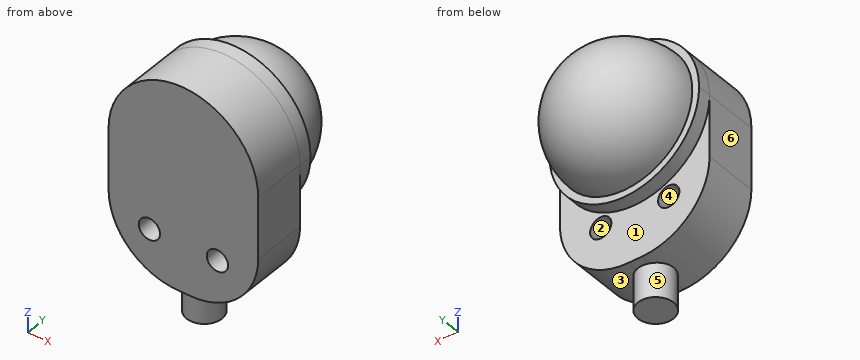
Autodesk Inventor part; units mm, degrees
ref_plane "Work Plane1" through (0, 0, 0) normal (1, 0, 0) x (0, 0, -1)
ref_plane "Work Plane2" through (0.5, 0, -9) normal (0, 0, -1) x (-1, 0, 0)
ref_plane "YZ Plane" through (0, 0, 0) normal (1, 0, 0) x (0, 1, 0)
sketch "Sketch1" plane through (0, 0, 0) normal (0, 1, 0) x (-1, 0, 0)
  arc A0 (5.5, 0) -> (-5.5, 0) centre (0, 0) ccw
  line L0 (5.5, 0) -> (5.5, -4.5)
  line L1 (-5.5, 0) -> (-5.5, -4.5)
  line L2 (-0.5, -9.5) -> (0.5, -9.5)
  arc A1 (-5.5, -4.5) -> (-0.5, -9.5) centre (-0.5, -4.5) ccw
  arc A2 (0.5, -9.5) -> (5.5, -4.5) centre (0.5, -4.5) ccw
  line L3 (0, 0) -> (0, -9.5) construction
  dimension "d0" = 11
  dimension "d1" = 15
  dimension "d2" = 5
extrude "Extrusion1" add sketch "Sketch1" along normal blind 4
sketch "Sketch2" plane through (0, 4, 0) normal (0, 1, 0) x (1, 0, 0)
  circle A0 centre (0, 0) radius 5.5
  arc A1 (-5.5, 0) -> (5.5, 0) centre (0, 0) ccw
extrude "Extrusion2" add sketch "Sketch2" along normal blind 1
ref_plane "Work Plane1" through (0, 0, 0) normal (1, 0, 0) x (0, 0, -1)
sketch "Sketch4" plane through (0, 0, 0) normal (1, 0, 0) x (0, 0, -1)
  line L0 (5.5, 5) -> (-5.5, 5)
  line L1 (0, 5) -> (0, 11.0328) construction
  arc A0 (5, 5) -> (0, 10) centre (0, 5) ccw
  line L2 (0, 10) -> (0, 5)
  line L3 (0, 5) -> (5, 5)
  point P0 (0, 0)
  dimension "d8" = 5
revolve "Revolution1" add sketch "Sketch4" angle 360 about axis through (0, 5, 0) along (0, 1, 0)
sketch "Sketch5" plane through (0, 0, 0) normal (0, -1, 0) x (1, 0, 0)
  line L0 (0, 0) -> (0, -9.4931) construction
  point P0 (2.5, -6)
  point P1 (-2.5, -6)
  dimension "d10" = 6
  dimension "d11" = 5
hole "Hole1" at (2.5, 0, -6) at (-2.5, 0, -6) direction (0, 1, 0) diameter 1.567 end through all
ref_plane "Work Plane2" through (0.5, 0, -9) normal (0, 0, -1) x (-1, 0, 0)
sketch "Sketch6" plane through (0.5, 0, -9) normal (0, 0, -1) x (-1, 0, 0)
  line L0 (0, 0) -> (1, 0)
  line L1 (1, 0) -> (1, 4)
  line L2 (0, 4) -> (1, 4)
  line L3 (0, 0) -> (0, 4)
  line L4 (0, 0) -> (0, 4)
  line L5 (0, 2) -> (1, 2) construction
  line L6 (1, 0) -> (1, 4)
  circle A0 centre (0.5, 2) radius 1.3
  point P0 (0.5, 0)
  dimension "d20" = 2.6
extrude "Extrusion3" add sketch "Sketch6" along normal blind 3 contours A0 L3 | L3 A0 L1 | L1 A0
properties part number "OptoForce_OMD-10-SE-10N"
Check sheet for the modelled part. Datum: model origin and axes. Units: mm. Face numbers are marked on the shaded views. A direction names the side the tool comes from. Give positions to 0.01 mm unless a question says otherwise; leave off trailing zeros. Loops run counter-clockwise (first coordinate to the right, second up) from the corner with the lowest first, then second, coordinate; pieces in that order, holes last. Notation, with made-up numbers: M 42.25,80.5 L 78.25,80.5 A20 cw 78.25,105.5 Z; hole C 72,21 d5. An arc over 180 degrees is marked long. Answer as a JSON object with one key per item and string values. Group by question number.
Q1. Go/stop test with flat-tipped pins: P1, Ø1.5, axis at x = 0.5, z = 1.5, coming from the +Y side; P2, Ø1, axis at y = 2, z = -5.5, coming from the +X side; P3, Ø0.6, axis at x = 0, y = 3.5, coming from the -Z side; P4, Ø1.4, axis at x = 2.5, z = -6, coming from the +Y side. Record where each tip stops, or that it passes through.
Q2. Cross-section at C-C on x = 0. Record the cut outline in (y, z), then the cut area to 3 significant figures.
Q3. Material ranges on line 1 along X through (y, z) = (0.5, -6); line 2 along Y through (x, z) = (3.25, 4); line 3 along Z through (x, y) = (2.5, 1.5), recorded low to high. Write a range as [from, to].
Q4. Cross-section at D-D on x = -2.5. Record the cut outline in (y, z).
Q5. Access from +Z, -Z, +X, -X, +Y, -Y to the whole of each face (thin tool, end or side, straight path). Record for the marked faces 5 and 6.
Q6. Release check for a two-part mould opening along X. For the marked faces 1, 2, 3 and 4 record: released by +X, released by -X, zero draft, split by the parting line, or undercut.
Q7. Cross-section at B-B on z = -6. Record the cut outline in (x, y).
Q8. Cross-section at A-A on y = 0.5. Record the cut outline in (x, z), then the cut area to 3 significant figures.
Evaluation:
{
 "1": {"P1": "stops at y = 9.93", "P2": "stops at x = 5.47", "P3": "stops at z = -12", "P4": "passes through"},
 "2": {"outline": "M 0,-9.5 L 0.7,-9.5 L 0.7,-12 L 3.3,-12 L 3.3,-9.5 L 4,-9.5 L 4,-5.5 L 5,-5.5 L 5,-5 A5 ccw 5,5 L 5,5.5 L 0,5.5 Z", "area": "117 mm2"},
 "3": {"line 1": "x = [-5.27, -3.28], [-1.72, 1.72], [3.28, 5.27]", "line 2": "y = [0, 5]", "line 3": "z = [-9.08, -6.78], [-5.22, 4.9]"},
 "4": {"outline": "M 0,-9.08 L 4,-9.08 L 4,-6.78 L 0,-6.78 Z; M 0,-5.22 L 4,-5.22 L 4,-4.9 L 5,-4.9 L 5,-4.33 A4.33 ccw 5,4.33 L 5,4.9 L 0,4.9 Z"},
 "5": {"face 5": "-Z", "face 6": "+Z, -Z, -X, +Y, -Y"},
 "6": {"face 1": "zero draft", "face 2": "undercut", "face 3": "released by +X", "face 4": "undercut"},
 "7": {"outline": "M -5.27,0 L -3.28,0 L -3.28,4 L -5.27,4 Z; M -1.72,0 L 1.72,0 L 1.72,4 L -1.72,4 Z; M 3.28,0 L 5.27,0 L 5.27,4 L 3.28,4 Z"},
 "8": {"outline": "M -5.5,-4.5 A5 ccw -0.5,-9.5 L 0.5,-9.5 A5 ccw 5.5,-4.5 L 5.5,0 A5.5 ccw -5.5,0 Z; hole C -2.5,-6 d1.57; hole C 2.5,-6 d1.57", "area": "137 mm2"}
}
